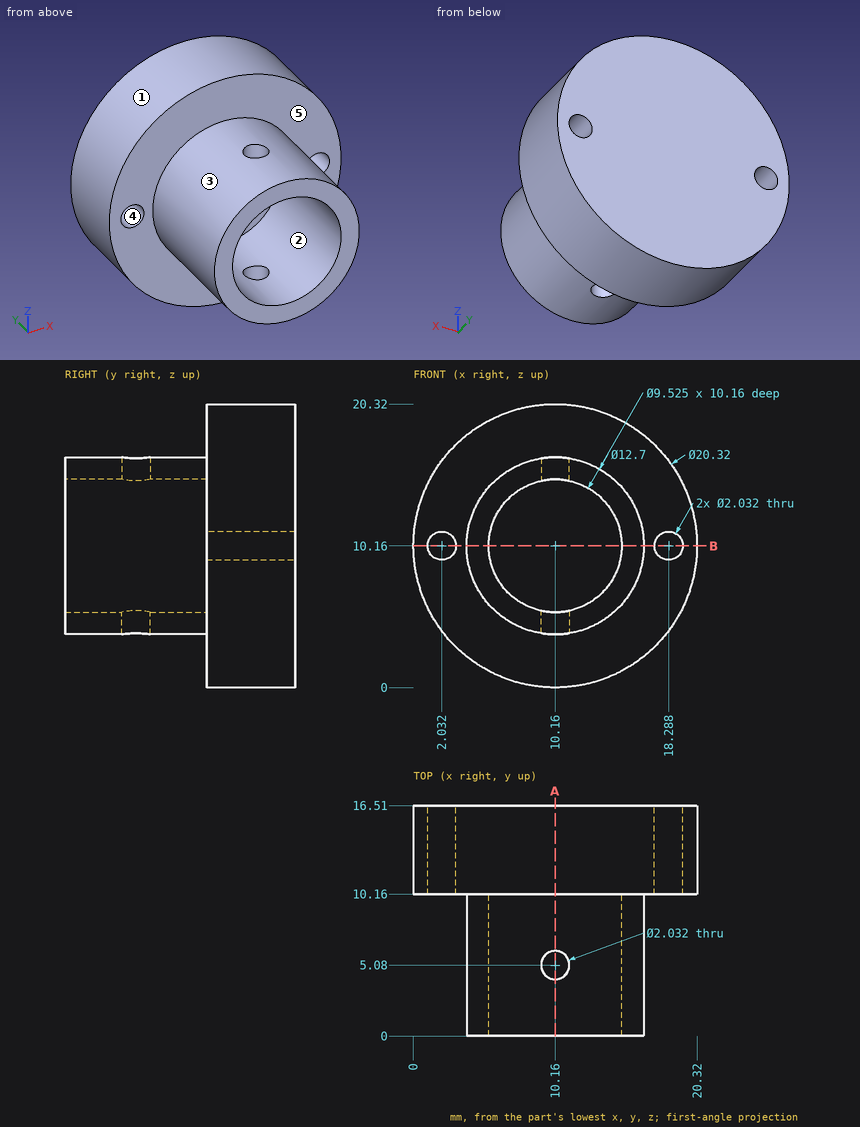
Input: dimensioned drawing with shaded views. Units: mm. Origin: part minimum x, y, z. A direction names the side the tool comes from. Round coordinates to 2 decimals unless told otherwise and drop trailing zeros. Loops run counter-clockwise (first coordinate to the right, second up) from the corner with the lowest first, then second, coordinate; pieces in that order, holes last. Notation, with made-up numbers: (55, 43.5) -> (89, 43.5) arc R24 cw to (89, 63.5) -> close; hole circle Ø9 at (-1.5, -35.75). An arc over 180 degrees is marked (long way). One line per item, written item: value.
(1) Mould query, pull axis Z, two halves, no side actions, for the marked faces 3, 4 and 5. Classes: pulls with the +Z half, pulls with the -Z half, needs draft (parallel to the pull), parting line crosses it, or undercut.
Geometry check:
face 3: parting line crosses it
face 4: undercut
face 5: needs draft
(2) Set-up query: the marked faces 1 and 2. Return all of +Z, -Z, +X, -X, +Y, -Y with unobstructed straight access to the full face (end or side cutting, diameter ignored); none if empty.
Geometry check:
face 1: +Y, -Y
face 2: -Y
(3) Pin query (flat end, axial travel): pin 1 (6 mm diameter, centred on x = 14.5, y = 3, fed in from -Z); pin 2 (5 mm diameter, centred on x = 9, y = 3.5, fed in from -Z); pin 3 (1.5 mm diameter, centred on y = 4.5, z = 6.5, fed in from +X); pin 4 (1.5 mm diameter, centred on x = 6.5, z = 13, fed in from -Y). Return the tip coordinate at first contact, or that it passes through.
Geometry check:
pin 1: z = 3.95
pin 2: z = 3.81
pin 3: x = 15.8
pin 4: y = 0
(4) Section B-B (z = 10.16). Return the cut outline in (x, y).
Geometry check:
outline: (0, 10.16) -> (1.02, 10.16) -> (1.02, 16.51) -> (0, 16.51) -> close; (3.05, 10.16) -> (3.81, 10.16) -> (3.81, 0) -> (5.4, 0) -> (5.4, 10.16) -> (14.92, 10.16) -> (14.92, 0) -> (16.51, 0) -> (16.51, 10.16) -> (17.27, 10.16) -> (17.27, 16.51) -> (3.05, 16.51) -> close; (19.3, 10.16) -> (20.32, 10.16) -> (20.32, 16.51) -> (19.3, 16.51) -> close
(5) Material intervals for line 1 (Y direction, x = 10.16, z = 16); line 2 (X direction, y = 14.25, z = 10.16); line 3 (Y direction, x = 13, z = 9), sorted ascending. Write a range as [from, to].
Geometry check:
line 1: [0, 4.06], [6.1, 16.51]
line 2: [0, 1.02], [3.05, 17.27], [19.3, 20.32]
line 3: [10.16, 16.51]
(6) Section A-A (x = 10.16). Return the cut outline in (y, z).
Geometry check:
outline: (0, 3.81) -> (4.06, 3.81) -> (4.06, 5.4) -> (0, 5.4) -> close; (0, 14.92) -> (4.06, 14.92) -> (4.06, 16.51) -> (0, 16.51) -> close; (6.1, 3.81) -> (10.16, 3.81) -> (10.16, 0) -> (16.51, 0) -> (16.51, 20.32) -> (10.16, 20.32) -> (10.16, 16.51) -> (6.1, 16.51) -> (6.1, 14.92) -> (10.16, 14.92) -> (10.16, 5.4) -> (6.1, 5.4) -> close
